```python
from build123d import *

# Parameters (mm, degrees)
BOSS_EXTRUDE1_DEPTH     = 30
SKETCH1_13_W            = 2
SKETCH1_13_H            = 12
BOSS_EXTRUDE6_DEPTH     = 30
CUT_EXTRUDE3_DEPTH      = 5
BOSS_EXTRUDE4_START     = -2.45
BOSS_EXTRUDE4_OUTLINE_W = 30
BOSS_EXTRUDE4_OUTLINE_H = 14.485281374
BOSS_EXTRUDE4_OUTLINE_R = 1.6
BOSS_EXTRUDE4_DEPTH     = 2.45
CUT_EXTRUDE1_DEPTH      = 5
SKETCH1_10_R            = 1.6
BOSS_EXTRUDE5_DEPTH     = 2.45
CUT_EXTRUDE4_DEPTH      = 63.353829072


# Read off the part's stored shape, not the designer's step: Boss-Extrude4
with BuildPart() as part:
    # Sketch1 → Boss-Extrude1 (new body)
    with BuildSketch(Plane.XY):
        Polygon((0, 12), (12, 0), (0, 0), align=None)
    boss_extrude1 = extrude(amount=BOSS_EXTRUDE1_DEPTH)

    # Sketch1<13> → Boss-Extrude6 (add)
    with BuildSketch(Plane.XY):
        with Locations((-1, 6)):
            Rectangle(SKETCH1_13_W, SKETCH1_13_H)
    boss_extrude6 = extrude(amount=BOSS_EXTRUDE6_DEPTH)

    # Sketch4 → Cut-Extrude3 (cut)
    with BuildSketch(Plane(origin=(6, 6, 0), x_dir=(0, 0, -1), z_dir=(0.7071067811865477, 0.7071067811865475, 0))):
        Polygon((-6.175, -8.485281374), (-6.175, 3.145733136), (-9, 4.776747647), (-11.825, 3.145733136), (-11.825, -8.485281374), align=None)
    cut_extrude3 = extrude(amount=-CUT_EXTRUDE3_DEPTH, mode=Mode.SUBTRACT)

    # Boss-Extrude4 outline → Boss-Extrude4 (add)
    with BuildSketch(Plane(origin=(6, 6, 0), x_dir=(0, 0, -1), z_dir=(0.7071067811865477, 0.7071067811865475, 0)).offset(BOSS_EXTRUDE4_START)):
        with Locations((-15, -1.242640687)):
            Rectangle(BOSS_EXTRUDE4_OUTLINE_W, BOSS_EXTRUDE4_OUTLINE_H)
        with Locations((-9, 1.514718626)):
            Circle(BOSS_EXTRUDE4_OUTLINE_R, mode=Mode.SUBTRACT)
    boss_extrude4 = extrude(amount=BOSS_EXTRUDE4_DEPTH)

    # Sketch1<4> → Cut-Extrude1 (cut)
    with BuildSketch(Plane.XY):
        Polygon((10.669337222, 0), (4.440608352, 6.623473909), (1.265296423, 5.876327682), (0.324688071, 2.752853773), (2.91347758, 0), align=None)
    cut_extrude1 = extrude(amount=CUT_EXTRUDE1_DEPTH, mode=Mode.SUBTRACT)

    # Sketch1<10> → Boss-Extrude5 (add)
    # profile 1 of 2: a face of its own
    with BuildSketch(Plane.XY):
        Polygon((2.559391648, 0.376526091), (5.734703577, 1.123672318), (6.675311929, 4.247146227), (4.440608352, 6.623473909), (1.265296423, 5.876327682), (0.324688071, 2.752853773), align=None)
        with Locations((3.5, 3.5)):
            Circle(SKETCH1_10_R, mode=Mode.SUBTRACT)
    # profile 2 of 2: a face of its own
    with BuildSketch(Plane.XY):
        Polygon((3.5, 0), (10.669337222, 0), (6.675311929, 4.247146227), (5.734703577, 1.123672318), (2.559391648, 0.376526091), (2.91347758, 0), align=None)
    boss_extrude5 = extrude(amount=BOSS_EXTRUDE5_DEPTH)

    # Mirror1: Boss-Extrude1, Boss-Extrude6, Cut-Extrude3, Boss-Extrude4, Cut-Extrude1, Boss-Extrude5 across plane
    add(boss_extrude1.mirror(Plane.XY.offset(30)))
    add(boss_extrude6.mirror(Plane.XY.offset(30)))
    add(cut_extrude3.mirror(Plane.XY.offset(30)), mode=Mode.SUBTRACT)
    add(boss_extrude4.mirror(Plane.XY.offset(30)))
    add(cut_extrude1.mirror(Plane.XY.offset(30)), mode=Mode.SUBTRACT)
    add(boss_extrude5.mirror(Plane.XY.offset(30)))

    # Sketch1<12> → Cut-Extrude4 (cut, through all)
    with BuildSketch(Plane.XY):
        Polygon((12, -3.5), (12, 0), (10.669337222, 0), (3.5, 0), (2.91347758, 0), (1.441458618, 0), (0, 0), (0, -3.5), align=None)
    extrude(amount=CUT_EXTRUDE4_DEPTH, mode=Mode.SUBTRACT)


solid = part.part
```
Could you check a few things on this model? Use its own coordinates, in mm. A direction names the side the tool comes from. Give positions to 0.01 mm unless a question says otherwise; leave off trailing zeros. Loops run counter-clockwise (first coordinate to the right, second up) from the corner with the lowest first, then second, coordinate; pieces in that order, holes last. Notation, with made-up numbers: (-22.75, -33.5) -> (26.25, -33.5) arc R30 ccw to (26.25, 2.5) -> close; hole circle Ø8 at (9, 8.25). An arc over 180 degrees is marked (long way). Put each result on its own line as item: value.
(1) For faces 1 (the face through (2, 5, 60)), 2 (the face through (-1, 12, 30)), 3 (the face through (5.509, 3.027, 8.96)), 4 (the face through (4.36, 4.85, 58.79)), 5 (the face through (7.599, 3.265, 3.707)), which set-ups out of +Z, -Z, +X, -X, +Y, -Y let a thin tool reach every point of the face, with its end or its side?
Computed:
face 1: +Z, +X, -X, +Y, -Y
face 2: +Z, -Z, +X, -X, +Y
face 3: none
face 4: +Z
face 5: -Y
(2) Imagine slicing it at A-A on y = 3.5. Write out the boundary of the cut face in (x, z) (3 decimals).
Computed:
outline: (-2, 0) -> (1.9, 0) -> (1.9, 2.45) -> (0.55, 2.45) -> (0.55, 5) -> (7.378, 5) -> (7.378, 2.45) -> (5.1, 2.45) -> (5.1, 0) -> (8.5, 0) -> (8.5, 60) -> (5.1, 60) -> (5.1, 57.55) -> (7.378, 57.55) -> (7.378, 55) -> (0.55, 55) -> (0.55, 57.55) -> (1.9, 57.55) -> (1.9, 60) -> (-2, 60) -> close; hole (1.429, 6.175) -> (5.035, 6.175) -> (5.035, 11.825) -> (1.429, 11.825) -> close; hole (1.429, 48.175) -> (5.035, 48.175) -> (5.035, 53.825) -> (1.429, 53.825) -> close
(3) Please list where these lines run through material, in increasing order: probe 1 along Z at (x, y) = (3.75, 4.75) (3 decimals); probe 2 along Z at (x, y) = (1.5, 2.25); probe 3 along Z at (x, y) = (4.5, 6). Write a range as [from, to].
Computed:
probe 1: [5, 6.175], [11.825, 48.175], [53.825, 55]
probe 2: [0, 2.45], [5, 55], [57.55, 60]
probe 3: [0, 2.45], [5, 7.47], [10.53, 49.47], [52.53, 55], [57.55, 60]
(4) Thinking about a two-plate mould opening in X: for faces 6 (the face through (2, 5, 0)), 7 (the face through (7.599, 3.265, 56.293)), which applies, pulls with the +X half, pulls with the -X half, needs draft (parallel to the pull), parting line crosses it, or undercut?
Computed:
face 6: needs draft
face 7: undercut
(5) Imagine slicing it at B-B on z = 25.5. Write out the boundary of the cut face in (x, y), plus the area to 3 significant figures.
Computed:
outline: (-2, 0) -> (12, 0) -> (0, 12) -> (-2, 12) -> close
area: 96.0 mm^2
(6) I'm going to push a flat-ended pin straight in: pin 1 Ø2 at (x, z) = (3, 21.5) entering from +Y. Where does the tip first touch, or does it pass through?
Computed:
pin 1: y = 10
(7) Imagine slicing it at D-D on x = 11.25. Write out the boundary of the cut face in (y, z).
Computed:
outline: (0, 0) -> (0.75, 0) -> (0.75, 60) -> (0, 60) -> close
